Here's the drawing with two shaded views (mm, measured from the low corner). I have some questions. Give positions to 0.01 mm unless a question says otherwise; leave off trailing zeros. Order: outer loops, then holes, each group sorted by start corner. A loop starts at its lowest first (then second) coordinate and runs counter-clockwise, first axis right, second up. Notation, with made-up numbers: (-13, 85.5) - (45, 85.5) arc R17 ccw to (45, 110.5) - close; hole circle Ø4 at (10, -9.5). An arc over 180 degrees is marked (long way). Use one line per item in the form item = value. Start each with the question number.
1) Suppose I cut it at A-A, the plane x = 120.5. Write out the boundary of the cut face in (y, z).
2) Please list where these lines run through material, in increasing order: probe 1 along Z at (x, y) = (6, 4); probe 2 along Z at (x, y) = (37.5, 9.75); probe 3 along X at (y, z) = (3, 182).
3) Suppose I cut it at C-C, the plane z = 196.5. Write out the boundary of the cut face in (x, y), and give its area (3 significant figures).
4) Suppose I cut it at B-B, the plane y = 2.75. Write out the boundary of the cut face in (x, z), and give its area (3 significant figures).
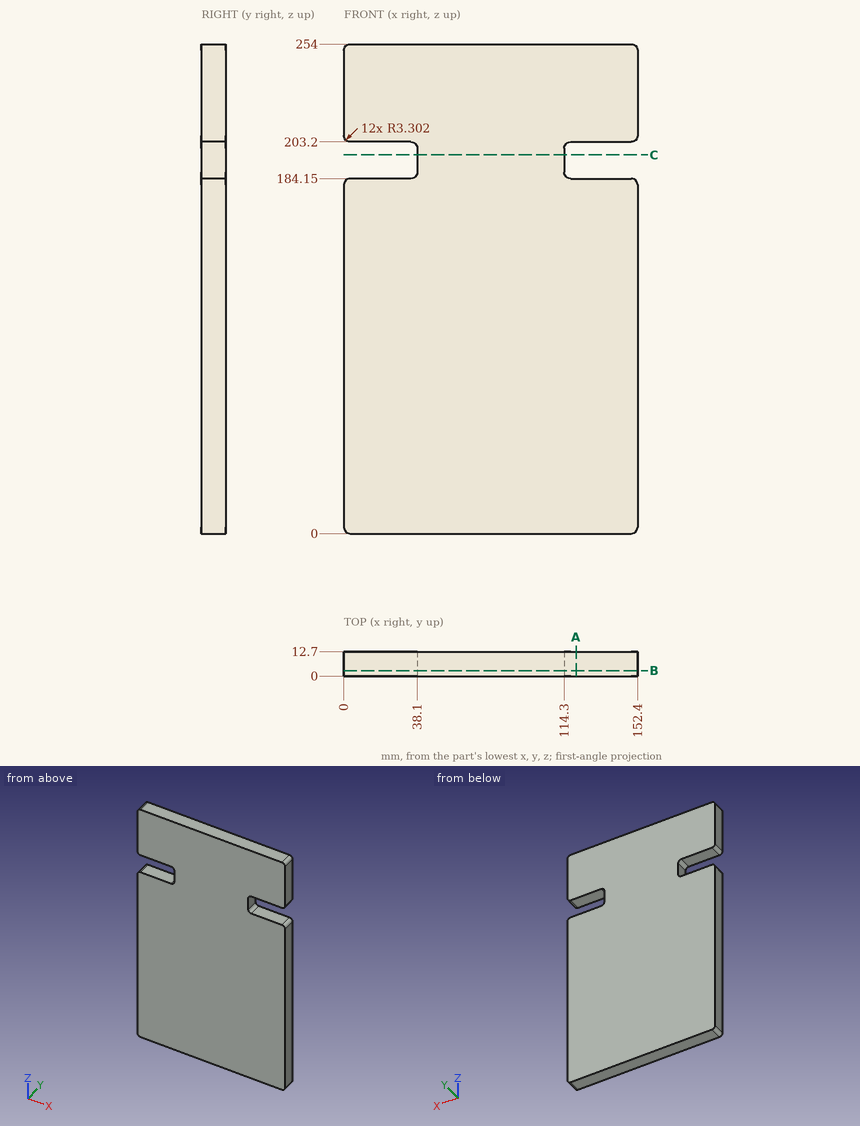
Result sheet:
q1.outline = (0, 0) - (12.7, 0) - (12.7, 184.15) - (0, 184.15) - close; (0, 203.2) - (12.7, 203.2) - (12.7, 254) - (0, 254) - close
q2.probe_1 = 0 to 184.15, 203.2 to 254
q2.probe_2 = 0 to 185.55, 201.8 to 254
q2.probe_3 = 0.21 to 152.19
q3.outline = (38.1, 0) - (114.3, 0) - (114.3, 12.7) - (38.1, 12.7) - close
q3.area = 968 mm²
q4.outline = (0, 3.3) arc R3.3 ccw to (3.3, 0) - (149.1, 0) arc R3.3 ccw to (152.4, 3.3) - (152.4, 180.85) arc R3.3 ccw to (149.1, 184.15) - (117.6, 184.15) arc R3.3 cw to (114.3, 187.45) - (114.3, 199.9) arc R3.3 cw to (117.6, 203.2) - (149.1, 203.2) arc R3.3 ccw to (152.4, 206.5) - (152.4, 250.7) arc R3.3 ccw to (149.1, 254) - (3.3, 254) arc R3.3 ccw to (0, 250.7) - (0, 206.5) arc R3.3 ccw to (3.3, 203.2) - (34.8, 203.2) arc R3.3 cw to (38.1, 199.9) - (38.1, 187.45) arc R3.3 cw to (34.8, 184.15) - (3.3, 184.15) arc R3.3 ccw to (0, 180.85) - close
q4.area = 37,200 mm²
